Could you check a few things on this model? Use its own coordinates, in mm. A direction names the side the tool comes from. Coordinates: 2 decimals unless noted, no trailing zeros. Loops run counter-clockwise (first coordinate to the right, second up) from the corner with the lowest first, then second, coordinate; pieces in that order, holes last. Notation, with made-up numbers: (-17, 15.25) -> (9, 15.25) arc R15 ccw to (9, 27.25) -> close; hole circle Ø3 at (-33.5, 48.25). An arc over 180 degrees is marked (long way). One line per question, with ' | ' between items.
from build123d import *

# Parameters (mm, degrees)
ESQUISSE1_W        = 30
ESQUISSE1_H        = 50
ESQUISSE1_R        = 14
ESQUISSE1_W_2      = 27
ESQUISSE1_H_2      = 18
BOSS_EXTRU_1_DEPTH = 1
ESQUISSE2_W        = 30
ESQUISSE2_H        = 21
ESQUISSE2_W_2      = 27
ESQUISSE2_H_2      = 18
BOSS_EXTRU_2_DEPTH = 2
CONG_1_R           = 1


with BuildPart() as part:
    # Esquisse1 → Boss.-Extru.1 (new body)
    with BuildSketch(Plane(origin=(0, 0, 0), x_dir=(1, 0, 0), z_dir=(0, 1, 0))):
        Rectangle(ESQUISSE1_W, ESQUISSE1_H)
        with Locations(Location((0, -10.5, 0), (0, 0, 270))):
            Circle(ESQUISSE1_R, mode=Mode.SUBTRACT)
        with Locations((0, 14.5)):
            Rectangle(ESQUISSE1_W_2, ESQUISSE1_H_2, mode=Mode.SUBTRACT)
    extrude(amount=BOSS_EXTRU_1_DEPTH)

    # Esquisse2 → Boss.-Extru.2 (add)
    with BuildSketch(Plane(origin=(0, 1, 0), x_dir=(1, 0, 0), z_dir=(0, 1, 0))):
        with Locations((0, 14.5)):
            Rectangle(ESQUISSE2_W, ESQUISSE2_H)
        with Locations((0, 14.5)):
            Rectangle(ESQUISSE2_W_2, ESQUISSE2_H_2, mode=Mode.SUBTRACT)
    extrude(amount=BOSS_EXTRU_2_DEPTH)

    # Congé1
    cong_1_edges = [part.edges().sort_by_distance(p)[0] for p in [
        (-15, 1.5, -25),
        (-15, 2, -4),
        (15, 1.5, -25),
        (15, 2, -4),
    ]]
    fillet(cong_1_edges, radius=CONG_1_R)


solid = part.part
1) If we section it at B-B on x = 0: Please give me the cut outline in (y, z).
Data:
outline: (0, -25) -> (3, -25) -> (3, -23.5) -> (0, -23.5) -> close; (0, -5.5) -> (3, -5.5) -> (3, -4) -> (1, -4) -> (1, -3.5) -> (0, -3.5) -> close; (0, 24.5) -> (1, 24.5) -> (1, 25) -> (0, 25) -> close
2) On a 3-axis mill with a long thin cutter (end or side, diameter ignored), from which of +Z, -Z, +X, -X, +Y, -Y can I reach the whole of each face in a straight line? I mean faces 1 (the face through (-14.715, 2.014, -4.301)), 2 (the face through (14.715, 2.014, -4.301)), 3 (the face through (13.5, 1, -14)). Say none if no direction works.
Data:
face 1: +Z, -X, +Y | face 2: +Z, +X, +Y | face 3: +Y, -Y
3) I need wall thicknesses on line 1 along Z through (x, y) = (-7, 1.05); line 2 along Z through (x, y) = (7, 0.4); line 3 along X through (y, z) = (2.75, -6.5). Which ranges of each line are inside material? Lowest first, please. Write a range as from..to.
Data:
line 1: -25..-23.5, -5.5..-4 | line 2: -25..-23.5, -5.5..-1.62, 22.62..25 | line 3: -15..-13.5, 13.5..15
4) I'm going to push a flat-ended pin straight in: pin 1 Ø0.9 at (x, y) = (-2, 2) entering from +Z. Where does the tip first touch, or does it pass through?
Data:
pin 1: z = -4
5) If we section it at D-D on x = -11: Please give me the cut outline in (y, z), and give its area (3 significant figures).
Data:
outline: (0, -25) -> (3, -25) -> (3, -23.5) -> (0, -23.5) -> close; (0, -5.5) -> (3, -5.5) -> (3, -4) -> (1, -4) -> (1, 1.84) -> (0, 1.84) -> close; (0, 19.16) -> (1, 19.16) -> (1, 25) -> (0, 25) -> close | area: 20.7 mm²
6) If we section it at C-C on y = 2.3: Please give me the cut outline in (x, z), and give its area (3 significant figures).
Data:
outline: (-15, -24) arc R1 ccw to (-14, -25) -> (14, -25) arc R1 ccw to (15, -24) -> (15, -5) arc R1 ccw to (14, -4) -> (-14, -4) arc R1 ccw to (-15, -5) -> close; hole (-13.5, -23.5) -> (13.5, -23.5) -> (13.5, -5.5) -> (-13.5, -5.5) -> close | area: 143 mm²
7) We'd pull the mould along Z, two halves only. Please class faces 4 (the face through (-14.715, 1.479, -24.699)), 5 (the face through (-0.2, 0.5, 25)), 6 (the face through (0, 1, -5.5)): pulls with the +Z half, pulls with the -Z half, needs draft (parallel to the pull), parting line crosses it, or undercut.
Data:
face 4: pulls with the -Z half | face 5: pulls with the +Z half | face 6: undercut
8) If we section it at A-A on z = 10.5: Please give me the cut outline in (x, y), and give its area (3 significant figures).
Data:
outline: (-15, 0) -> (-14, 0) -> (-14, 1) -> (-15, 1) -> close; (14, 0) -> (15, 0) -> (15, 1) -> (14, 1) -> close | area: 2.00 mm²
